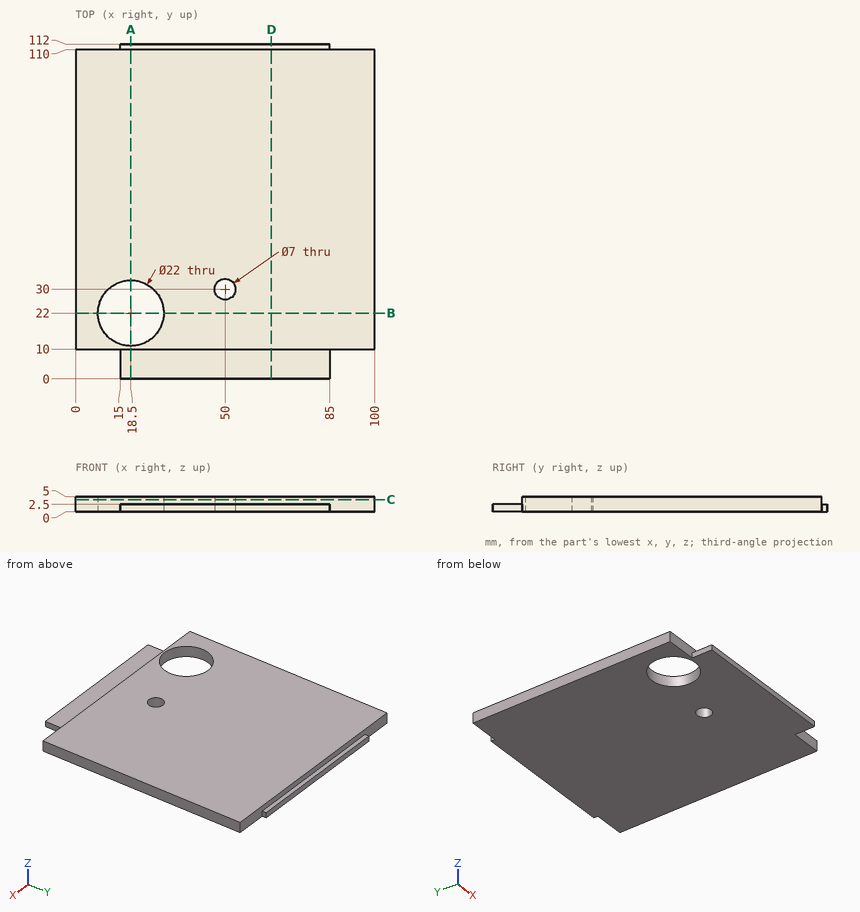
Check sheet for the drawn part. Datum: minimum x, y, z corner. Units: mm. Round coordinates to 2 decimals unless told otherwise and drop trailing zeros. Order: outer loops, then holes, each group sorted by start corner. A loop starts at its lowest first (then second) coordinate and runs counter-clockwise, first axis right, second up. Notation, with made-up numbers: M -0.5,-19.5 L 25.5,-19.5 A20 cw 25.5,8.5 Z; hole C -10,54.25 d2. An arc over 180 degrees is marked long. Answer in a Markdown table with one row per item.
(1) Section check D-D on x = 65.5. Record the boundary of the cut face in (y, z).
Findings:
| item | result |
|---|---|
| outline | M 0,0 L 112,0 L 112,2.5 L 110,2.5 L 110,5 L 10,5 L 10,2.5 L 0,2.5 Z |
(2) Gauge pin test, flat ends, axial feed: pin 1 (2 mm diameter, centred on y = 6, z = 1.5, fed in from -X); pin 2 (4 mm diameter, centred on x = 50, y = 30, fed in from -Z); pin 3 (0.6 mm diameter, centred on x = 33.5, y = 111.5, fed in from +Z); pin 4 (1.2 mm diameter, centred on y = 4.5, z = 0.5, fed in from +X). Record the tip position at first contact, or that the pin passes through.
Findings:
| item | result |
|---|---|
| pin 1 | stops at x = 15 |
| pin 2 | passes through |
| pin 3 | stops at z = 2.5 |
| pin 4 | stops at x = 85 |
(3) Section check C-C on z = 4.1. Record the boundary of the cut face in (x, y), plus the area to 3 significant figures.
Findings:
| item | result |
|---|---|
| outline | M 0,10 L 100,10 L 100,110 L 0,110 Z; hole C 18.5,22 d22; hole C 50,30 d7 |
| area | 9,580 mm^2 |
(4) Section check A-A on x = 18.5. Record the boundary of the cut face in (y, z), plus the area to 3 significant figures.
Findings:
| item | result |
|---|---|
| outline | M 0,0 L 11,0 L 11,5 L 10,5 L 10,2.5 L 0,2.5 Z; M 33,0 L 112,0 L 112,2.5 L 110,2.5 L 110,5 L 33,5 Z |
| area | 420 mm^2 |
(5) Section check B-B on y = 22. Record the boundary of the cut face in (x, z), plus the area to 3 significant figures.
Findings:
| item | result |
|---|---|
| outline | M 0,0 L 7.5,0 L 7.5,5 L 0,5 Z; M 29.5,0 L 100,0 L 100,5 L 29.5,5 Z |
| area | 390 mm^2 |
(6) Material ranges on line 1 along Y through (x, z) = (18.5, 3.3); line 2 along Y through (x, z) = (50, 3.7); line 3 along X through (y, z) = (30, 2.9), recorded low to high. Write a range as from..to.
Findings:
| item | result |
|---|---|
| line 1 | y = 10..11, 33..110 |
| line 2 | y = 10..26.5, 33.5..110 |
| line 3 | x = 0..10.95, 26.05..46.5, 53.5..100 |
